Could you check a few things on this model? Use its own coordinates, in mm. A direction names the side the tool comes from. Coordinates: 2 decimals unless noted, no trailing zeros. Order: outer loops, then holes, each group sorted by start corner. A loop starts at its lowest first (then second) coordinate and runs counter-clockwise, first axis right, second up. Notation, with made-up numbers: (73.5, 28) -> (107.5, 28) arc R16 cw to (107.5, 36) -> close; hole circle Ø9 at (11.5, 42.5). An arc over 180 degrees is marked (long way). Use a Markdown table: item, result. Add a question column.
1) Thinking about a two-plate mould opening in X: for faces 1 (the flat face through (-5, -5, -65)), 2 (the flat face through (-6, -6, -92)), 3 (the flat face through (2, -3, 67.5)), which applies, +X half, -X half, draft (parallel to the pull), parting line (faces both ways), or undercut?
2) If we section it at B-B (z = 42): Write out the boundary of the cut face in (x, y).
3) If we section it at C-C (x = 41): Write out the boundary of the cut face in (y, z).
4) Will these pins go through, and if not, where does the flat tip stop? pin 1 Ø1.8 at (x, y) = (19, -8) entering from +Z; pin 2 Ø5 at (y, z) = (0, -96) entering from +X; pin 3 Ø4.5 at (y, z) = (-3.5, -81) entering from -X.
5) If we section it at A-A (x = 0): Write out the boundary of the cut face in (y, z).
6) Which directions (+Z, -Z, +X, -X, +Y, -Y) give clear straight access to the entire face, cutting with the end or side of a thin tool? Please do faces 4 (the flat face through (-9, -6, -96.1)), 5 (the flat face through (-9, -6, -85.3)), 6 (the flat face through (20, -6, -79.875)), 7 (the flat face through (-2, -3, -67.3)), 8 (the flat face through (17, -6, -97)).
7) If I drill on L1, parallel to Y at x = 39, z = -55; L2, parallel to X at y = -9, z = 64.5; L3, parallel to X at y = -3.75, z = -63.5, over which ranges is the centre line in solid material (lowest first)? Write a range as [from, to].
```python
from build123d import *

# Parameters (mm, degrees)
F0_W     = 6
F0_H     = 5.4244026542
F0_H_2   = 17
F0_H_3   = 8
F0_W_2   = 10
F0_H_4   = 3.5826090725
F1_DEPTH = 5
F2_DEPTH = 12.5
F3_DEPTH = 10
F5_D     = 5
F5_DEPTH = 105.1006789719
F6_D     = 5
F7_D     = 3


with BuildPart() as f1:
    # F0 (on Front) → F1 (new body)
    with BuildSketch(Plane.XZ):
        with BuildLine():
            ThreePointArc((5, 62.2996789719), (45.9279326772, 42.3895623945), (62.5, 0))
            ThreePointArc((62.5, 0), (45.9279326772, -42.3895623945), (5, -62.2996789719))
            Line((5, -62.2996789719), (5, -63.7170698994))
            Line((5, -63.7170698994), (23, -63.7170698994))
            Line((23, -63.7170698994), (23, -74.008445464))
            ThreePointArc((23, -74.008445464), (62.40492769, -45.9551411705), (77.5, 0))
            ThreePointArc((77.5, 0), (-50.3798074629, 58.8907887534), (-12, -76.5653315803))
            Line((-12, -76.5653315803), (-12, -63.7170698994))
            Line((-12, -63.7170698994), (-5, -63.7170698994))
            Line((-5, -63.7170698994), (-5, -62.2996789719))
            ThreePointArc((-5, -62.2996789719), (-62.5, 0), (-5, 62.2996789719))
            Line((-5, 62.2996789719), (-5, 67.5))
            Line((-5, 67.5), (5, 67.5))
            Line((5, 67.5), (5, 62.2996789719))
        make_face()
        with BuildLine():
            Line((23, -79.8752763177), (23, -74.008445464))
            ThreePointArc((23, -74.008445464), (5.6466287865, -77.2940203596), (-12, -76.5653315803))
            Line((-12, -76.5653315803), (-12, -79.8752763177))
            Line((-12, -79.8752763177), (-6, -79.8752763177))
            Line((-6, -79.8752763177), (-6, -85.2996789719))
            Line((-6, -85.2996789719), (-12, -85.2996789719))
            Line((-12, -85.2996789719), (-12, -88.0996789719))
            Line((-12, -88.0996789719), (-6, -88.0996789719))
            Line((-6, -88.0996789719), (-6, -96.0996789719))
            Line((-6, -96.0996789719), (-12, -96.0996789719))
            Line((-12, -96.0996789719), (-12, -105.0996789719))
            Line((-12, -105.0996789719), (17, -105.0996789719))
            Line((17, -105.0996789719), (17, -88.0996789719))
            Line((17, -88.0996789719), (23, -88.0996789719))
            Line((23, -88.0996789719), (23, -85.2996789719))
            Line((23, -85.2996789719), (17, -85.2996789719))
            Line((17, -85.2996789719), (17, -79.8752763177))
            Line((17, -79.8752763177), (23, -79.8752763177))
        make_face()
        with BuildLine():
            Line((23, -63.7170698994), (5, -63.7170698994))
            Line((5, -63.7170698994), (5, -67.2996789719))
            Line((5, -67.2996789719), (-5, -67.2996789719))
            Line((-5, -67.2996789719), (-5, -63.7170698994))
            Line((-5, -63.7170698994), (-12, -63.7170698994))
            Line((-12, -63.7170698994), (-12, -76.5653315803))
            ThreePointArc((-12, -76.5653315803), (5.6466287865, -77.2940203596), (23, -74.008445464))
            Line((23, -74.008445464), (23, -63.7170698994))
        make_face()
        with Locations((20, -82.5874776448)):
            Rectangle(F0_W, F0_H)
        with Locations((20, -96.5996789719)):
            Rectangle(F0_W, F0_H_2)
        with Locations((-9, -82.5874776448)):
            Rectangle(F0_W, F0_H)
        with Locations((-9, -92.0996789719)):
            Rectangle(F0_W, F0_H_3)
        with Locations((0, -65.5083744356)):
            Rectangle(F0_W_2, F0_H_4)
        with BuildLine():
            Line((5, -63.7170698994), (5, -62.2996789719))
            ThreePointArc((5, -62.2996789719), (0, -62.5), (-5, -62.2996789719))
            Line((-5, -62.2996789719), (-5, -63.7170698994))
            Line((-5, -63.7170698994), (5, -63.7170698994))
        make_face()
        with BuildLine():
            ThreePointArc((-5, 62.2996789719), (0, 62.5), (5, 62.2996789719))
            Line((5, 62.2996789719), (5, 67.5))
            Line((5, 67.5), (-5, 67.5))
            Line((-5, 67.5), (-5, 62.2996789719))
        make_face()
    extrude(amount=-F1_DEPTH)

    # F0 (on Front) → F2 (join)
    with BuildSketch(Plane.XZ):
        with Locations((20, -82.5874776448)):
            Rectangle(F0_W, F0_H)
        with Locations((20, -96.5996789719)):
            Rectangle(F0_W, F0_H_2)
        with Locations((-9, -92.0996789719)):
            Rectangle(F0_W, F0_H_3)
        with Locations((-9, -82.5874776448)):
            Rectangle(F0_W, F0_H)
    extrude(amount=F2_DEPTH)

    # F0 (on Front) → F3 (join)
    with BuildSketch(Plane.XZ):
        with BuildLine():
            ThreePointArc((-5, 62.2996789719), (0, 62.5), (5, 62.2996789719))
            Line((5, 62.2996789719), (5, 67.5))
            Line((5, 67.5), (-5, 67.5))
            Line((-5, 67.5), (-5, 62.2996789719))
        make_face()
        with BuildLine():
            Line((5, -63.7170698994), (5, -62.2996789719))
            ThreePointArc((5, -62.2996789719), (0, -62.5), (-5, -62.2996789719))
            Line((-5, -62.2996789719), (-5, -63.7170698994))
            Line((-5, -63.7170698994), (5, -63.7170698994))
        make_face()
        with Locations((0, -65.5083744356)):
            Rectangle(F0_W_2, F0_H_4)
    extrude(amount=F3_DEPTH)

    # F5 (through all, one way)
    with BuildSketch(Plane.XY):
        with Locations((0, -5)):
            Circle(F5_D / 2)
    extrude(amount=-F5_DEPTH, mode=Mode.SUBTRACT)

    # F6 (through all)
    with Locations(Plane(origin=(0, 0, 0), x_dir=(1, 0, 0), z_dir=(0, 0, -1))):
        with Locations((0, 5)):
            Hole(F6_D / 2)

    # F7 (through all)
    with Locations(Plane.XZ):
        with Locations((-70, 0), (70, 0)):
            Hole(F7_D / 2)


solid = f1.part
```
Answer sheet:
| question | item | result |
|---|---|---|
| 1 | face 1 | -X half |
| 1 | face 2 | undercut |
| 1 | face 3 | draft |
| 2 | outline | (-65.13, 0) -> (-46.28, 0) -> (-46.28, 5) -> (-65.13, 5) -> close; (46.28, 0) -> (65.13, 0) -> (65.13, 5) -> (46.28, 5) -> close |
| 3 | outline | (0, -65.77) -> (5, -65.77) -> (5, -47.17) -> (0, -47.17) -> close; (0, 47.17) -> (5, 47.17) -> (5, 65.77) -> (0, 65.77) -> close |
| 4 | pin 1 | z = -79.88 |
| 4 | pin 2 | x = 23 |
| 4 | pin 3 | x = -12 |
| 5 | outline | (-10, -67.3) -> (-7.5, -67.3) -> (-7.5, -62.5) -> (-10, -62.5) -> close; (-10, 62.5) -> (-7.5, 62.5) -> (-7.5, 67.5) -> (-10, 67.5) -> close; (-2.5, -67.3) -> (0, -67.3) -> (0, -105.1) -> (5, -105.1) -> (5, -62.5) -> (-2.5, -62.5) -> close; (-2.5, 62.5) -> (5, 62.5) -> (5, 77.5) -> (0, 77.5) -> (0, 67.5) -> (-2.5, 67.5) -> close |
| 6 | face 4 | -Z, -X, -Y |
| 6 | face 5 | +X, -X, -Y |
| 6 | face 6 | +Z, +X, -X, -Y |
| 6 | face 7 | -Z, +X, -X, -Y |
| 6 | face 8 | +Z, -Z, -Y |
| 7 | L1 | [0, 5] |
| 7 | L2 | [-5, 5] |
| 7 | L3 | [-5, -2.17], [2.17, 5] |
